Can you work these out from the drawing? Everything is in mm from the part's minimum corner. A direction names the side the tool comes from. Coordinates: 2 decimals unless noted, no trailing zeros. Order: outer loops, then holes, each group sorted by start corner. A loop starts at its lowest first (then second) coordinate and runs counter-clockwise, first axis right, second up. Notation, with made-up numbers: (41.5, 84) -> (45.5, 84) arc R12 ccw to (45.5, 99) -> close; hole circle Ø2 at (79, 31). An arc over 180 degrees is marked (long way). Use a Markdown table: item, result. Add a question column.
1) Which directions (+Z, -Z, +X, -X, +Y, -Y) give clear straight access to the entire face, cutting with the end or side of a thin tool? Please do the marked faces 1, 2, 3 and 4.
2) If I drill on L1, parallel to Z at x = 5.25, y = 2.5; L2, parallel to Y at x = 13.5, z = 15.75, over which ranges is the centre line in solid material (lowest first)? Write a range as [from, to].
3) If we section it at D-D (y = 16.75): Write out the boundary of the cut face in (x, z).
4) If we section it at C-C (z = 11.75): Write out the boundary of the cut face in (x, y).
5) Will these pins go through, and if not, where does the flat tip stop? pin 1 Ø3 at (y, z) = (8, 17) entering from +X; pin 2 Ø3 at (y, z) = (10, 15.5) entering from -X; pin 3 Ø6 at (x, z) = (11, 10) entering from -Y; pin 4 Ø5 at (x, z) = (12, 15.5) entering from +Y.
6) If we section it at A-A (x = 6): Write out the boundary of the cut face in (y, z), plus the area to 3 significant figures.
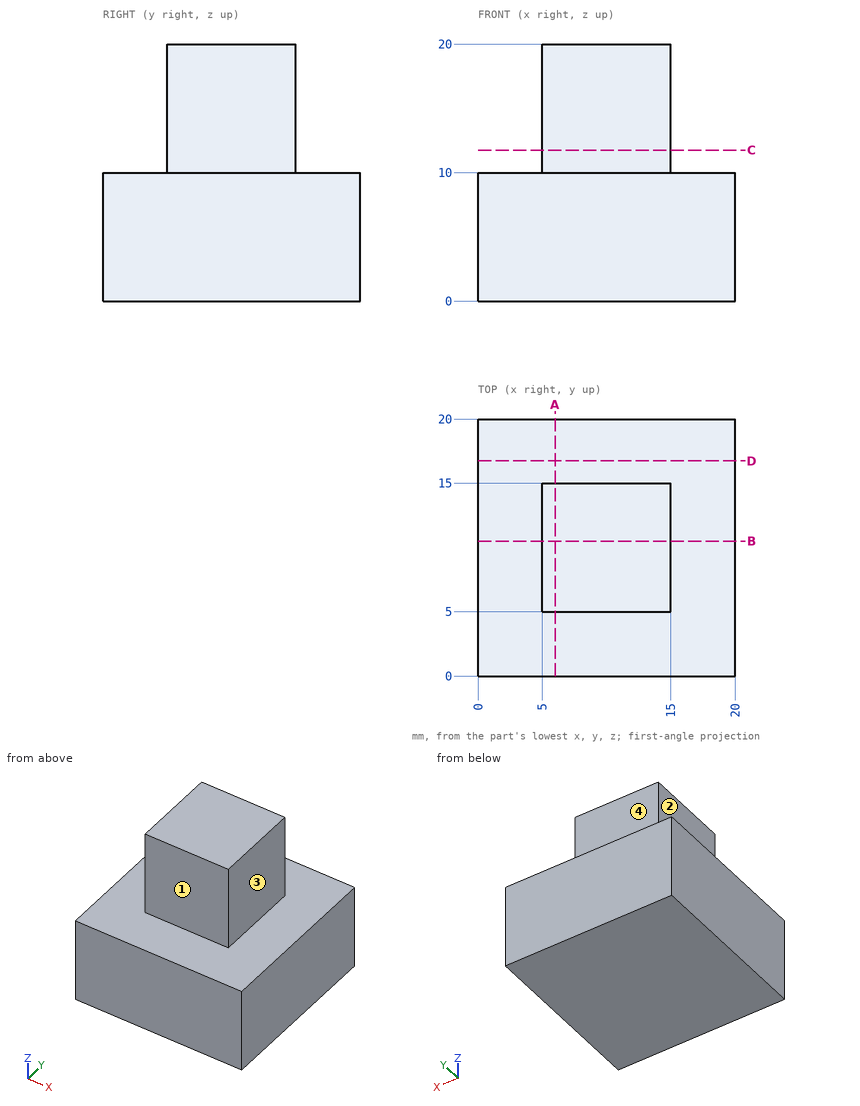
Answer sheet:
| question | item | result |
|---|---|---|
| 1 | face 1 | +Z, +X, -X, -Y |
| 1 | face 2 | +Z, -X, +Y, -Y |
| 1 | face 3 | +Z, +X, +Y, -Y |
| 1 | face 4 | +Z, +X, -X, +Y |
| 2 | L1 | [0, 10] |
| 2 | L2 | [5, 15] |
| 3 | outline | (0, 0) -> (20, 0) -> (20, 10) -> (0, 10) -> close |
| 4 | outline | (5, 5) -> (15, 5) -> (15, 15) -> (5, 15) -> close |
| 5 | pin 1 | x = 15 |
| 5 | pin 2 | x = 5 |
| 5 | pin 3 | y = 0 |
| 5 | pin 4 | y = 15 |
| 6 | outline | (0, 0) -> (20, 0) -> (20, 10) -> (15, 10) -> (15, 20) -> (5, 20) -> (5, 10) -> (0, 10) -> close |
| 6 | area | 300 mm2 |
